from build123d import *

# Parameters (mm, degrees)
SKETCH073_R     = 3
SKETCH073_W     = 2.3
SKETCH073_H     = 7.3
PAD053_DEPTH    = 2
CHAMFER_SIZE    = 1.9
CHAMFER006_SIZE = 1.9


with BuildPart() as part:
    # Sketch073 → Pad053 (new body)
    with BuildSketch(Plane.YZ.offset(31.5)):
        Polygon((8, 0), (4, 6.928203), (-4, 6.928203), (-8, 0), (-4, -6.928203), (-4, -20), (4, -20), (4, -6.928203), align=None)
        Circle(SKETCH073_R, mode=Mode.SUBTRACT)
        with Locations((0, -13.5)):
            Rectangle(SKETCH073_W, SKETCH073_H, mode=Mode.SUBTRACT)
    extrude(amount=PAD053_DEPTH)

    # Chamfer
    chamfer_edges = [part.edges().sort_by_distance(p)[0] for p in [
        (33.5, -6, 3.464102),
        (33.5, -6, -3.464102),
        (33.5, 0, 6.928203),
        (33.5, 6, 3.464102),
        (33.5, 6, -3.464102),
    ]]
    chamfer(chamfer_edges, length=CHAMFER_SIZE)

    # Chamfer006
    chamfer006_edges = [part.edges().sort_by_distance(p)[0] for p in [
        (33.5, 0, -20),
    ]]
    chamfer(chamfer006_edges, length=CHAMFER006_SIZE)


solid = part.part
Can you work these out from the model? Positions are in its coordinate system, mm. A direction names the side the tool comes from. Round coordinates to 2 decimals unless told otherwise and drop trailing zeros. Order: outer loops, then holes, each group sorted by start corner. A loop starts at its lowest first (then second) coordinate and runs counter-clockwise, first axis right, second up. Notation, with made-up numbers: (-18.5, -37) - (17.5, -37) arc R9 cw to (17.5, -30) - close; hole circle Ø2 at (87.25, 54.5). An arc over 180 degrees is marked (long way). Answer in a Markdown table with one row per item.
(1) Suppose I cut it at D-D, the plane z = 1. Please give me the cut outline in (x, y), plus the area to 3 significant figures.
From the geometry:
| item | result |
|---|---|
| outline | (31.5, -7.42) - (31.6, -7.42) - (33.5, -5.23) - (33.5, -2.83) - (31.5, -2.83) - close; (31.5, 2.83) - (33.5, 2.83) - (33.5, 5.23) - (31.6, 7.42) - (31.5, 7.42) - close |
| area | 14.2 mm2 |
(2) Suppose I cut it at A-A, the plane z = -16. Please give me the cut outline in (x, y), plus the area to 3 significant figures.
From the geometry:
| item | result |
|---|---|
| outline | (31.5, -4) - (33.5, -4) - (33.5, -1.15) - (31.5, -1.15) - close; (31.5, 1.15) - (33.5, 1.15) - (33.5, 4) - (31.5, 4) - close |
| area | 11.4 mm2 |
(3) If we mould it in two halves opening along Y, with no side actions, what happens to faces 4 (the face through (32, -3, 0)), 5 (the face through (33.5, 0, -6)), 6 (the face through (32, -4, -11))? For each: released by +Y, released by -Y, zero draft, split by the parting line, or undercut.
From the geometry:
| item | result |
|---|---|
| face 4 | undercut |
| face 5 | zero draft |
| face 6 | released by -Y |
(4) Suppose I cut it at B-B, the plane x = 33.05. Please give me the cut outline in (y, z), plus the area to 3 significant figures.
From the geometry:
| item | result |
|---|---|
| outline | (-6.33, 0) - (-4, -4.03) - (-4, -18.55) - (4, -18.55) - (4, -4.03) - (6.33, 0) - (3.16, 5.48) - (-3.16, 5.48) - close; hole circle Ø6 at (0, 0); hole (-1.15, -17.15) - (1.15, -17.15) - (1.15, -9.85) - (-1.15, -9.85) - close |
| area | 165 mm2 |
(5) Please list where these lines run through material, in increasing order: L1, parallel to Z at x = 32.05, y = 0; L2, parallel to Z at x = 32.3, y = 0; L3, parallel to Y at x = 32.25, z = -12.75. Write a range as from..to.
From the geometry:
| item | result |
|---|---|
| L1 | z = -19.55..-17.15, -9.85..-3, 3..6.48 |
| L2 | z = -19.3..-17.15, -9.85..-3, 3..6.23 |
| L3 | y = -4..-1.15, 1.15..4 |
(6) For P1, Ø0.6, axis at x = 32.5, z = -13.5, coming from the +Y side; P2, Ø0.6, axis at x = 32.5, z = -7.5, coming from the -Y side; P3, Ø0.6, axis at x = 33, y = 0, coming from the -Z side, each with a flat end and sliding along its axis, tell me the tip position at first contact or that it passes through.
From the geometry:
| item | result |
|---|---|
| P1 | stops at y = 4 |
| P2 | stops at y = -4 |
| P3 | stops at z = -18.9 |
(7) Suppose I cut it at C-C, the plane y = -3.5. Please give me the cut outline in (x, z).
From the geometry:
| item | result |
|---|---|
| outline | (31.5, -20) - (31.6, -20) - (33.5, -18.1) - (33.5, 3.99) - (32.47, 6.06) - (31.6, 6.93) - (31.5, 6.93) - close |
(8) Which directions (+Z, -Z, +X, -X, +Y, -Y) give clear straight access to the entire face, cutting with the end or side of a thin tool? Please do faces 1 (the face through (32.35, -5.38, -3.04)), 2 (the face through (32, 1.15, -14)), 3 (the face through (32, 4, -12)).
From the geometry:
| item | result |
|---|---|
| face 1 | -Z, +X, -Y |
| face 2 | +X, -X |
| face 3 | -Z, +X, +Y |
